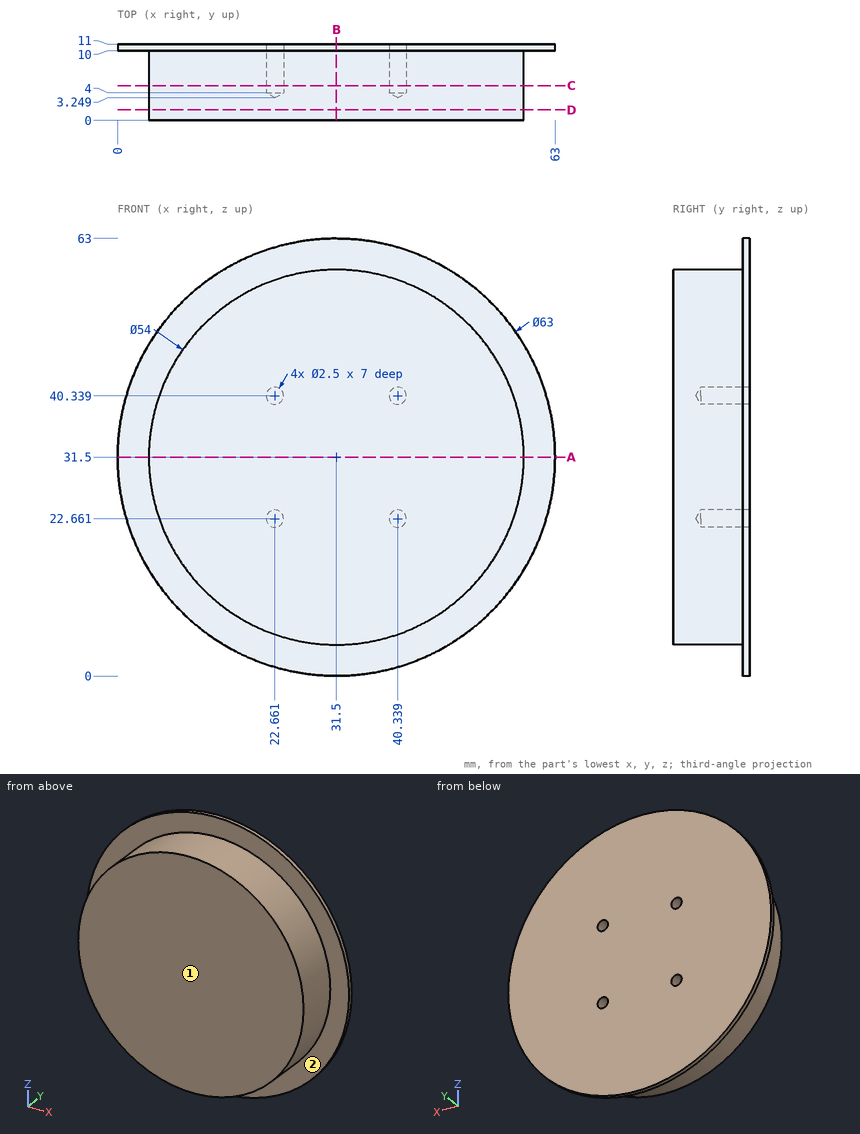
The figure shows three views and two pictorial views of one solid part (mm, origin at its lowest corner). Answer the questions. A direction names the side the tool comes from. Round coordinates to 2 decimals unless told otherwise and drop trailing zeros. Write each loop counter-clockwise with the first axis right and the second up, starting at its lowest first coordinate (ties: lowest second). Pieces come first, ordered by that corner, then holes. Notation, with made-up numbers: M 59.25,-36.75 L 98.25,-36.75 A17 cw 98.25,-30.75 Z; hole C 13.25,70 d10. An arc over 180 degrees is marked long. Use a Markdown table: item, result.
1) The part is cut by section C-C on y = 5. Give the vertices of the cut face in (x, z), plus the area to 3 significant figures.
Taken from the geometry:
| item | result |
|---|---|
| outline | C 31.5,31.5 d54; hole C 22.66,22.66 d2.5; hole C 22.66,40.34 d2.5; hole C 40.34,22.66 d2.5; hole C 40.34,40.34 d2.5 |
| area | 2,270 mm2 |
2) Consider line 1 (X direction, y = 10.25, z = 40); line 2 (Z direction, x = 22, y = 6.5); line 3 (Y direction, x = 6, z = 16.5). Determine where each line is inside the solid, lowest interval first. Write a range as [from, to].
Taken from the geometry:
| item | result |
|---|---|
| line 1 | x = [1.17, 21.46], [23.86, 39.14], [41.54, 61.83] |
| line 2 | z = [6.23, 21.6], [23.72, 39.28], [41.4, 56.77] |
| line 3 | y = [10, 11] |
3) The part is cut by section B-B on x = 31.5. Give the vertices of the cut face in (y, z).
Taken from the geometry:
| item | result |
|---|---|
| outline | M 0,4.5 L 10,4.5 L 10,0 L 11,0 L 11,63 L 10,63 L 10,58.5 L 0,58.5 Z |
4) The part is cut by section A-A on z = 31.5. Give the vertices of the cut face in (x, y), plus the area to 3 significant figures.
Taken from the geometry:
| item | result |
|---|---|
| outline | M 0,10 L 4.5,10 L 4.5,0 L 58.5,0 L 58.5,10 L 63,10 L 63,11 L 0,11 Z |
| area | 603 mm2 |
5) Flat-ended cylindrical pins translate along their axes: pin 1 (3 mm diameter, centred on x = 35, y = 1.5, fed in from +Z); pin 2 (1 mm diameter, centred on y = 7, z = 41.5, fed in from +X); pin 3 (6 mm diameter, centred on y = 2.5, z = 15, fed in from -X). Find the tip coordinate at first contact, or state that the pin passes through.
Taken from the geometry:
| item | result |
|---|---|
| pin 1 | stops at z = 58.43 |
| pin 2 | stops at x = 56.77 |
| pin 3 | stops at x = 8.12 |
6) The part is cut by section D-D on y = 1.5. Give the vertices of the cut face in (x, z).
Taken from the geometry:
| item | result |
|---|---|
| outline | C 31.5,31.5 d54 |
7) Which of the six approach directions +Z, -Z, +X, -X, +Y, -Y give full straight-line access (tool end or side, diameter ignored) to the marked faces 1 and 2?
Taken from the geometry:
| item | result |
|---|---|
| face 1 | +Z, -Z, +X, -X, -Y |
| face 2 | -Y |
